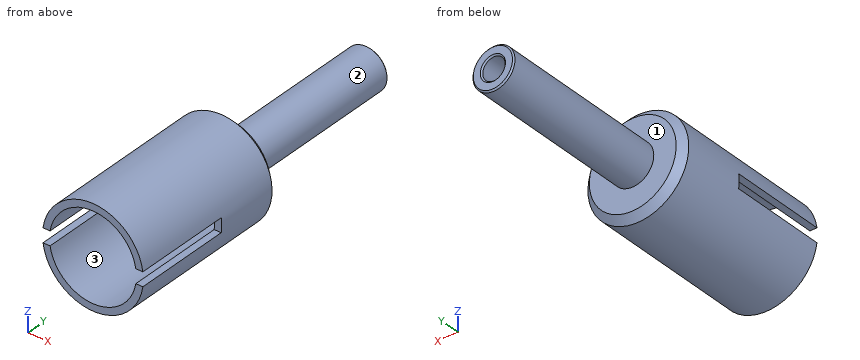
from build123d import *

# Parameters (mm, degrees)
SCHIZZO1_R        = 36
ESTRUSIONE1_DEPTH = 120
SCHIZZO2_R        = 31
ESTRUSIONE2_DEPTH = 110
SMUSSO1_SIZE      = 5
SCHIZZO3_R        = 15
ESTRUSIONE3_DEPTH = 125
SCHIZZO4_R        = 8
ESTRUSIONE4_DEPTH = 251.23389059
SMUSSO2_SIZE      = 1
SCHIZZO5_W        = 88.337421072
SCHIZZO5_H        = 10
ESTRUSIONE5_DEPTH = 70


with BuildPart() as part:
    # Schizzo1 → Estrusione1 (new body)
    with BuildSketch(Plane(origin=(0, 0, 0), x_dir=(1, 0, 0), z_dir=(0, 1, 0))):
        with Locations(Location((0, 0, 0), (0, 0, 270))):
            Circle(SCHIZZO1_R)
    extrude(amount=ESTRUSIONE1_DEPTH)

    # Schizzo2 → Estrusione2 (cut)
    with BuildSketch(Plane.XZ):
        with Locations(Location((0, 0, 0), (0, 0, 270))):
            Circle(SCHIZZO2_R)
    extrude(amount=-ESTRUSIONE2_DEPTH, mode=Mode.SUBTRACT)

    # Smusso1
    smusso1_edges = [part.edges().sort_by_distance(p)[0] for p in [
        (0, 120, -36),
    ]]
    chamfer(smusso1_edges, length=SMUSSO1_SIZE)

    # Schizzo3 → Estrusione3 (add)
    with BuildSketch(Plane(origin=(0, 120, 0), x_dir=(1, 0, 0), z_dir=(0, 1, 0))):
        with Locations(Location((0, 0, 0), (0, 0, 270))):
            Circle(SCHIZZO3_R)
    extrude(amount=ESTRUSIONE3_DEPTH)

    # Schizzo4 → Estrusione4 (cut, through all)
    with BuildSketch(Plane(origin=(0, 245, 0), x_dir=(1, 0, 0), z_dir=(0, 1, 0))):
        with Locations(Location((0, 0, 0), (0, 0, 270))):
            Circle(SCHIZZO4_R)
    extrude(amount=-ESTRUSIONE4_DEPTH, mode=Mode.SUBTRACT)

    # Smusso2
    smusso2_edges = [part.edges().sort_by_distance(p)[0] for p in [
        (0, 245, -15),
        (0, 245, -8),
    ]]
    chamfer(smusso2_edges, length=SMUSSO2_SIZE)

    # Schizzo5 → Estrusione5 (cut)
    with BuildSketch(Plane.XZ):
        Rectangle(SCHIZZO5_W, SCHIZZO5_H)
    extrude(amount=-ESTRUSIONE5_DEPTH, mode=Mode.SUBTRACT)


solid = part.part
Work out the finished part from the listing and answer in its coordinate system (mm). Face numbers are marked on the shaded views. Round coordinates to 2 decimals unless told otherwise and drop trailing zeros. Write each loop counter-clockwise with the first axis right and the second up, starting at its lowest first coordinate (ties: lowest second). Pieces come first, ordered by that corner, then holes. Notation, with made-up numbers: (67, 25) -> (75, 25) arc R23 cw to (75, 52) -> close; hole circle Ø2 at (-2, 85). An arc over 180 degrees is marked (long way). Answer as CSV lines item,"result". Start each with the question number.
(1) The part is cut by section D-D, the plane y = 185.5. Give the vertices of the cut face in (x, z), then the cut area to 3 significant figures.
(2) The part is cut by section C-C, the plane y = 25. Give the vertices of the cut face in (x, z).
(3) Find the intervals of material crossed by probe 1 along X at (y, z) = (72.5, 0); probe 2 along X at (y, z) = (168, 0); probe 3 along Y at (x, z) = (16.5, 8), in increasing order.
(4) The part is cut by section B-B, the plane z = 0. Give the vertices of the cut face in (x, y).
(5) Each of these flat-tipped pins is pushed along its axis until it touches: pin 1 (4.5 mm diameter, centred on x = -33, z = -0.5, fed in from -Y); pin 2 (10 mm diameter, centred on x = -9, y = 195, fed in from +Z); pin 3 (4 mm diameter, centred on x = 32, y = 45, fed in from -Z); pin 4 (18.5 mm diameter, centred on x = -4, z = -3.5, fed in from +Y). Where does it stop, or does it pass through?
(6) The mould has two halves that part along X. Classify the marked faces 1, 2 and 3: +X half, -X half, draft (parallel to the pull), parting line (faces both ways), or undercut.
(7) The part is cut by section A-A, the plane x = 0. Give the vertices of the cut face in (y, z).
Output values:
1,outline,"circle Ø30 at (0, 0); hole circle Ø16 at (0, 0)"
1,area,"506 mm²"
2,outline,"(-35.65, -5) arc R36 ccw to (35.65, -5) -> (30.59, -5) arc R31 cw to (-30.59, -5) -> close; (-35.65, 5) -> (-30.59, 5) arc R31 cw to (30.59, 5) -> (35.65, 5) arc R36 ccw to start"
3,probe 1,"x = -36 to -31, 31 to 36"
3,probe 2,"x = -15 to -8, 8 to 15"
3,probe 3,"y = 110 to 120"
4,outline,"(-36, 70) -> (-31, 70) -> (-31, 110) -> (-8, 110) -> (-8, 244) -> (-9, 245) -> (-14, 245) -> (-15, 244) -> (-15, 120) -> (-31, 120) -> (-36, 115) -> close; (8, 110) -> (31, 110) -> (31, 70) -> (36, 70) -> (36, 115) -> (31, 120) -> (15, 120) -> (15, 244) -> (14, 245) -> (9, 245) -> (8, 244) -> close"
5,pin 1,"stops at y = 70"
5,pin 2,"stops at z = 14.46"
5,pin 3,"stops at z = -19.9"
5,pin 4,"stops at y = 245"
6,face 1,"draft"
6,face 2,"parting line"
6,face 3,"undercut"
7,outline,"(0, -36) -> (115, -36) -> (120, -31) -> (120, -15) -> (244, -15) -> (245, -14) -> (245, -9) -> (244, -8) -> (110, -8) -> (110, -31) -> (0, -31) -> close; (0, 31) -> (110, 31) -> (110, 8) -> (244, 8) -> (245, 9) -> (245, 14) -> (244, 15) -> (120, 15) -> (120, 31) -> (115, 36) -> (0, 36) -> close"
